Build history of the part. All positions in model axes, mm. Face numbers are marked on the shaded views. A direction names the side the tool comes from. Round coordinates to 2 decimals unless told otherwise and drop trailing zeros. Write each loop counter-clockwise with the first axis right and the second up, starting at its lowest first coordinate (ties: lowest second). Pieces come first, ordered by that corner, then holes. Notation, with made-up numbers: (51.25, 41) -> (93.25, 41) arc R25 cw to (93.25, 77) -> close; hole circle Ø9 at (38, 29). An arc over 180 degrees is marked (long way). One line per question, with ' | ' between items.
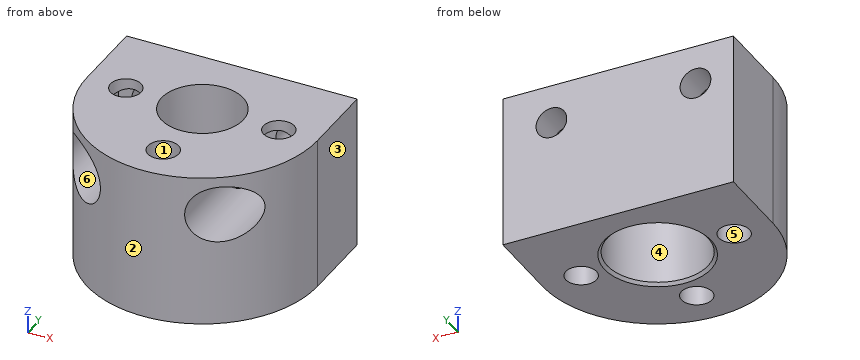
from build123d import *

# Parameters (mm, degrees)
RESSALTO_EXTRUS_O1_DEPTH                = 10
RESSALTO_EXTRUS_O1_DEPTH_BACK           = 6
ESBO_O2_R                               = 5.25
CORTE_EXTRUS_O1_DEPTH                   = 16
CORTE_EXTRUS_O1_DEPTH_BACK              = 31.8
M3_CLEARANCE_HOLE5_D                    = 3.2
CBORE_FOR_M5_HEX_HEAD_BOLT1_D           = 3.2
CBORE_FOR_M5_HEX_HEAD_BOLT1_CBORE_D     = 6
CBORE_FOR_M5_HEX_HEAD_BOLT1_CBORE_DEPTH = 16.5
SKETCH11_W                              = 24
SKETCH11_H                              = 16
SKETCH11_R                              = 1.6
BOSS_EXTRUDE3_DEPTH                     = 1
SKETCH12_R                              = 5.25
SKETCH12_R_2                            = 4.25
BOSS_EXTRUDE5_DEPTH                     = 6
CHAMFER1_SIZE                           = 0.3
SKETCH13_R                              = 3
CUT_EXTRUDE1_DEPTH                      = 43.8


with BuildPart() as part:
    # Esboço1 → Ressalto-extrusão1 (new body, two sides)
    with BuildSketch(Plane.XY) as ressalto_extrus_o1_sk:
        with BuildLine():
            Line((115.646593224, -302.7659332), (115.646593224, -295.7159332))
            Line((115.646593224, -295.7159332), (91.646593224, -295.7159332))
            Line((91.646593224, -295.7159332), (91.646593224, -302.7659332))
            ThreePointArc((91.646593224, -302.7659332), (103.646593224, -314.7659332), (115.646593224, -302.7659332))
        make_face()
    extrude(amount=RESSALTO_EXTRUS_O1_DEPTH)
    extrude(ressalto_extrus_o1_sk.sketch, amount=-RESSALTO_EXTRUS_O1_DEPTH_BACK)

    # Esboço2 → Corte-extrusão1 (cut, two sides)
    with BuildSketch(Plane.XY.offset(10)) as corte_extrus_o1_sk:
        with Locations((103.646593224, -302.7659332)):
            Circle(ESBO_O2_R)
    extrude(amount=CORTE_EXTRUS_O1_DEPTH, mode=Mode.SUBTRACT)
    extrude(corte_extrus_o1_sk.sketch, amount=-CORTE_EXTRUS_O1_DEPTH_BACK, mode=Mode.SUBTRACT)

    # M3 Clearance Hole5 (through all)
    with Locations(Plane.XY.offset(10)):
        with Locations((95.681870132, -302.765933199), (103.646593224, -310.730656291), (111.611316315, -302.765933199)):
            Hole(M3_CLEARANCE_HOLE5_D / 2)

    # CBORE for M5 Hex Head Bolt1 (through all)
    with Locations(Plane(origin=(0, -314.7159332, 0), x_dir=(-1, 0, 0), z_dir=(0, -1, 0))):
        with Locations((-95.596593224, -5.949346208), (-110.596593224, -5.949346208)):
            CounterBoreHole(CBORE_FOR_M5_HEX_HEAD_BOLT1_D / 2, CBORE_FOR_M5_HEX_HEAD_BOLT1_CBORE_D / 2, CBORE_FOR_M5_HEX_HEAD_BOLT1_CBORE_DEPTH)

    # Sketch11 → Boss-Extrude3 (add)
    with BuildSketch(Plane(origin=(0, -295.7159332, 0), x_dir=(1, 0, 0), z_dir=(0, 1, 0))):
        with Locations((103.646593224, -2)):
            Rectangle(SKETCH11_W, SKETCH11_H)
        with Locations((95.596593224, -5.949346208)):
            Circle(SKETCH11_R, mode=Mode.SUBTRACT)
        with Locations((110.596593224, -5.949346208)):
            Circle(SKETCH11_R, mode=Mode.SUBTRACT)
    extrude(amount=BOSS_EXTRUDE3_DEPTH)

    # Sketch12 → Boss-Extrude5 (add)
    with BuildSketch(Plane.XY.offset(10)):
        with Locations((103.646593224, -302.7659332)):
            Circle(SKETCH12_R)
        with Locations((103.646593224, -302.7659332)):
            Circle(SKETCH12_R_2, mode=Mode.SUBTRACT)
    extrude(amount=-BOSS_EXTRUDE5_DEPTH)

    # Chamfer1
    chamfer1_edges = [part.edges().sort_by_distance(p)[0] for p in [
        (98.396593224, -302.7659332, -6),
    ]]
    chamfer(chamfer1_edges, length=CHAMFER1_SIZE)

    # Sketch13 → Cut-Extrude1 (cut)
    with BuildSketch(Plane.XZ.offset(298.2159332)):
        with Locations((95.596593224, 5.949346208)):
            Circle(SKETCH13_R)
        with Locations((110.596593224, 5.949346208)):
            Circle(SKETCH13_R)
    extrude(amount=CUT_EXTRUDE1_DEPTH, mode=Mode.SUBTRACT)


solid = part.part
(1) Mould opens along X. For the marked faces 1, 2 and 3 say: pulls with the +X half, pulls with the -X half, needs draft (parallel to the pull), parting line crosses it, or undercut.
Calculated:
face 1: undercut | face 2: parting line crosses it | face 3: pulls with the +X half
(2) Wall check: line 1 (Y direction, x = 103.5, z = -5.5); line 2 (X direction, y = -302.75, z = 1.5); line 3 (X direction, y = -305.5, z = 8.5). Give the ranges that are in metal, low to high. Write a range as from..to.
Calculated:
line 1: -314.77..-312.32, -309.14..-308.01, -297.52..-294.72 | line 2: 91.65..94.08, 97.28..98.4, 108.9..110.01, 113.21..115.65 | line 3: 91.96..94.02, 97.18..100.39, 106.9..109.02, 112.18..115.33
(3) Slice it at D-D (z = 1). Write the cut outline in (x, y), then the cut area to 3 significant figures.
Calculated:
outline: (91.65, -302.77) arc R12 ccw to (115.65, -302.77) -> (115.65, -294.72) -> (91.65, -294.72) -> close; hole circle Ø3.2 at (95.68, -302.77); hole circle Ø10.5 at (103.65, -302.77); hole circle Ø3.2 at (103.65, -310.73); hole circle Ø3.2 at (111.61, -302.77) | area: 309 mm2
(4) Slice it at A-A (z = 6.5). Write the cut outline in (x, y).
Calculated:
outline: (91.65, -302.77) arc R12 ccw to (92.65, -307.56) -> (92.65, -298.22) -> (94.09, -298.22) -> (94.09, -294.72) -> (91.65, -294.72) -> close; (97.1, -298.22) -> (98.55, -298.22) -> (98.55, -313.63) arc R12 ccw to (107.65, -314.08) -> (107.65, -304.2) arc R4.25 cw (long way) to (107.65, -301.33) -> (107.65, -298.22) -> (109.09, -298.22) -> (109.09, -294.72) -> (97.1, -294.72) -> close; (112.1, -298.22) -> (113.55, -298.22) -> (113.55, -309.55) arc R12 ccw to (115.65, -302.77) -> (115.65, -294.72) -> (112.1, -294.72) -> close; hole circle Ø3.2 at (103.65, -310.73)
(5) Slice it at C-C (x = 111.75). Write the cut outline in (y, z), then the cut area to 3 significant figures.
Calculated:
outline: (-311.62, -6) -> (-304.36, -6) -> (-304.36, 3.18) -> (-311.62, 3.18) -> close; (-311.62, 8.72) -> (-304.36, 8.72) -> (-304.36, 10) -> (-311.62, 10) -> close; (-301.17, -6) -> (-294.72, -6) -> (-294.72, 4.84) -> (-298.22, 4.84) -> (-298.22, 3.18) -> (-301.17, 3.18) -> close; (-301.17, 8.72) -> (-298.22, 8.72) -> (-298.22, 7.06) -> (-294.72, 7.06) -> (-294.72, 10) -> (-301.17, 10) -> close | area: 155 mm2
(6) 3-axis set-ups, long thin cutter, end or side, ignore diameter. For the marked faces 4, 5 and 6: which of +Z, -Z, +X, -X, +Y, -Y reach the whole face in a straight line?
Calculated:
face 4: -Z | face 5: +Z, -Z | face 6: -Y
(7) Drop flat-ended pins along their axis: pin 1 (4 mm diameter, centred on x = 111.61, y = -302.77, fed in from -Z); pin 2 (3 mm diameter, centred on y = -304.5, z = 7.5, fed in from +X); pin 3 (1 mm diameter, centred on y = -311, z = 4, fed in from -X); pin 4 (6.5 mm diameter, centred on x = 110.5, z = 6, fed in from -Y). Give the stop position or say it passes through.
Calculated:
pin 1: z = -6 | pin 2: x = 115.64 | pin 3: x = 97.33 | pin 4: y = -314.21
(8) Slice it at B-B (y = -310). Write the cut outline in (x, z).
Calculated:
outline: (94.07, -6) -> (102.22, -6) -> (102.22, 10) -> (94.07, 10) -> (94.07, 8.53) arc R3 cw (long way) to (94.07, 3.37) -> close; (105.07, -6) -> (113.22, -6) -> (113.22, 4.5) arc R3 cw (long way) to (113.22, 7.4) -> (113.22, 10) -> (105.07, 10) -> close
